from build123d import *

# Parameters (mm, degrees)
SKETCH1_W           = 14.6
SKETCH1_H           = 14.6
BOSS_EXTRUDE1_DEPTH = 1.5
SKETCH2_W           = 5.8
SKETCH2_H           = 3.2
SKETCH2_W_2         = 3.2
SKETCH2_H_2         = 5.8
BOSS_EXTRUDE2_DEPTH = 1.5
SKETCH4_W           = 14.6
SKETCH4_H           = 13
BOSS_EXTRUDE3_DEPTH = 3
FILLET5_R           = 3
CHAMFER1_SIZE       = 3
FILLET4_R           = 2


with BuildPart() as part:
    # Sketch1 → Boss-Extrude1 (new, symmetric)
    with BuildSketch(Plane(origin=(0, 0, 0), x_dir=(1, 0, 0), z_dir=(0, 1, 0))):
        Rectangle(SKETCH1_W, SKETCH1_H)
    extrude(amount=BOSS_EXTRUDE1_DEPTH, both=True)

    # Sketch2 → Boss-Extrude2 (add, symmetric)
    with BuildSketch(Plane(origin=(0, 0, 0), x_dir=(1, 0, 0), z_dir=(0, 1, 0))):
        with Locations((0, 8.9)):
            Rectangle(SKETCH2_W, SKETCH2_H)
        with Locations((0, -8.9)):
            Rectangle(SKETCH2_W, SKETCH2_H)
        with Locations((-8.9, 0)):
            Rectangle(SKETCH2_W_2, SKETCH2_H_2)
        with Locations((8.9, 0)):
            Rectangle(SKETCH2_W_2, SKETCH2_H_2)
    extrude(amount=BOSS_EXTRUDE2_DEPTH, both=True)

    # Sketch4 → Boss-Extrude3 (add)
    with BuildSketch(Plane.ZY.offset(10.5)):
        with Locations((0, -5)):
            Rectangle(SKETCH4_W, SKETCH4_H)
    boss_extrude3 = extrude(amount=BOSS_EXTRUDE3_DEPTH)

    # Mirror1: Boss-Extrude3 across plane
    add(boss_extrude3.mirror(Plane(origin=(0, 0, 0), x_dir=(0, 0, 1), z_dir=(1, 0, 0))))

    # Fillet5
    fillet5_edges = [part.edges().sort_by_distance(p)[0] for p in [
        (-13.5, 1.5, 0),
        (13.5, 1.5, 0),
    ]]
    fillet(fillet5_edges, radius=FILLET5_R)

    # Chamfer1
    chamfer1_edges = [part.edges().sort_by_distance(p)[0] for p in [
        (13.5, -11.5, 0),
        (-13.5, -11.5, 0),
    ]]
    chamfer(chamfer1_edges, length=CHAMFER1_SIZE - 0.0001)  # a hair under: the kernel refuses the full size

    # Fillet4
    fillet4_edges = [part.edges().sort_by_distance(p)[0] for p in [
        (-12.00005, -10.00005, 7.3),
        (-12.00005, -10.00005, -7.3),
        (12.00005, -10.00005, 7.3),
        (12.00005, -10.00005, -7.3),
    ]]
    fillet(fillet4_edges, radius=FILLET4_R)


solid = part.part
Can you work these out from the model? Positions are in its coordinate system, mm. A direction names the side the tool comes from. Coordinates: 2 decimals unless noted, no trailing zeros. Loops run counter-clockwise (first coordinate to the right, second up) from the corner with the lowest first, then second, coordinate; pieces in that order, holes last. Notation, with made-up numbers: (18, 62) - (49, 62) arc R12 cw to (49, 78) - close; hole circle Ø2 at (38.25, 73.25). An arc over 180 degrees is marked (long way). Answer as a JSON object with one key per item and string values. Group by question number.
Item 1: If I drill on L1, parallel to X at y = -4.5, z = -4.75; L2, parallel to Z at x = 8, y = -1; L3, parallel to Y at x = 2.5, z = 5.5, over which ranges is the centre line in solid material (lowest first)? Write a range as from..to.
Item 2: If we section it at D-D (y = 0.5): List the corners of the cut face in (x, z) for me, plus the area to 3 significant figures.
Item 3: For pin 1 (1 mm diameter, centred on x = -4.5, z = 4, fed in from -Y); pin 2 (0.9 mm diameter, centred on x = -9.5, y = 0.5, fed in from -Z); pin 3 (3.5 mm diameter, centred on x = 9.5, y = 0, fed in from -Z); pin 4 (2.5 mm diameter, centred on y = -0.5, z = 4.5, fed in from -X), each with a flat end and sliding along its axis, tell me the tip position at first contact or that it passes through.
Item 4: If we section it at B-B (z = -3.5): State how many separate pieces and enclosed holes the cut face has, plus the area to 3 significant figures.
Item 5: If we section it at C-C (x = 0): List the corners of the cut face in (y, z) for me, plus the area to 3 significant figures.
Item 6: If we section it at A-A (y = -3.5): List the corners of the cut face in (x, z) for me.
Item 7: On a 3-axis mill with a long thin cutter (end or side, diameter ignored), from which of +Z, -Z, +X, -X, +Y, -Y can I reach the whole of each face in a straight line? I mean faces 1 (the face through (-7.3, 0, -5)), 2 (the face through (-2.9, 0, 9)), 3 (the face through (5, 0, -7.3)), 4 (the face through (-5, 0, -7.3)). Say none if no direction works.
Returned:
{
 "1": {"L1": "x = -13.5..-10.5, 10.5..13.5", "L2": "z = -2.9..2.9", "L3": "y = -1.5..1.5"},
 "2": {"outline": "(-12.74, -7.3) - (-10.5, -7.3) - (-10.5, -2.9) - (-7.3, -2.9) - (-7.3, -7.3) - (-2.9, -7.3) - (-2.9, -10.5) - (2.9, -10.5) - (2.9, -7.3) - (7.3, -7.3) - (7.3, -2.9) - (10.5, -2.9) - (10.5, -7.3) - (12.74, -7.3) - (12.74, 7.3) - (10.5, 7.3) - (10.5, 2.9) - (7.3, 2.9) - (7.3, 7.3) - (2.9, 7.3) - (2.9, 10.5) - (-2.9, 10.5) - (-2.9, 7.3) - (-7.3, 7.3) - (-7.3, 2.9) - (-10.5, 2.9) - (-10.5, 7.3) - (-12.74, 7.3) - close", "area": "353 mm²"},
 "3": {"pin 1": "stops at y = -1.5", "pin 2": "stops at z = -2.9", "pin 3": "stops at z = -7.3", "pin 4": "stops at x = -13.5"},
 "4": {"separate pieces": "3", "enclosed holes": "0", "area": "109 mm²"},
 "5": {"outline": "(-1.5, -10.5) - (1.5, -10.5) - (1.5, 10.5) - (-1.5, 10.5) - close", "area": "63.0 mm²"},
 "6": {"outline": "(-13.5, -7.3) - (-10.5, -7.3) - (-10.5, 7.3) - (-13.5, 7.3) - close; (10.5, -7.3) - (13.5, -7.3) - (13.5, 7.3) - (10.5, 7.3) - close"},
 "7": {"face 1": "-Z, +Y, -Y", "face 2": "+Z, -X, +Y, -Y", "face 3": "-Z, +X, +Y, -Y", "face 4": "-Z, -X, +Y, -Y"}
}
